```python
from build123d import *

# Parameters (mm, degrees)
F0_W     = 18
F0_H     = 18
F1_DEPTH = 2
F3_D     = 2.54
F5_D     = 2.54


with BuildPart() as f1:
    # F0 (on Top) → F1 (new body)
    with BuildSketch(Plane.XY):
        Rectangle(F0_W, F0_H)
    extrude(amount=F1_DEPTH)

    # F3 (through all)
    with Locations(Plane.XY.offset(2)):
        with Locations((6.7902, 6.7902)):
            Hole(F3_D / 2)

    # F5 (through all)
    with Locations(Plane(origin=(0, 0, 0), x_dir=(1, 0, 0), z_dir=(0, 0, -1))):
        with Locations((-6.7902, -6.7902)):
            Hole(F5_D / 2)


solid = f1.part
```
Model file for the job. Use its own axes, mm. Coordinates: 2 decimals unless noted, no trailing zeros. Loops run counter-clockwise (first coordinate to the right, second up) from the corner with the lowest first, then second, coordinate; pieces in that order, holes last. Notation, with made-up numbers: M -33,58 L -26,58 A35 ccw -26,90 Z; hole C -40,68 d9. An arc over 180 degrees is marked long. Use CSV: the item, a comma, the result in double quotes. Start each with the question number.
1. Band-saw the part on B-B, the plane z = 1.65. List the corners of the cut face in (x, y), then the cut area to 3 significant figures.
2. Flat gauge pin, fed straight in: pin 1 (2 mm diameter, centred on x = 6.79, y = 6.79, fed in from -Z). Where does the tip first touch, or does it go through?
3. Band-saw the part on A-A, the plane y = 7.75. List the corners of the cut face in (x, z).
4. Probe probe 1 along Y at (x, z) = (-6.75, 1.3); probe 2 along Y at (x, z) = (7.25, 1.45); probe 3 along X at (y, z) = (6.5, 0.7). List the from-to ranges inside material, lowest first. Write a range as [from, to].
5. Two-plate mould, pull along X, no slides. Class faces 1 (the cylindrical face through (-7.376, 7.917, 1.014)), 2 (the cylindrical face through (6.107, 7.861, 0.986)), 3 (the flat face through (0, 0, 2)), 4 (the flat face through (-9, 0, 1)): pulls with the +X half, pulls with the -X half, needs draft (parallel to the pull), parting line crosses it, or undercut.
Entries:
1,outline,"M -9,-9 L 9,-9 L 9,9 L -9,9 Z; hole C -6.79,6.79 d2.54; hole C 6.79,6.79 d2.54"
1,area,"314 mm2"
2,pin 1,"passes through"
3,outline,"M -9,0 L -7.62,0 L -7.62,2 L -9,2 Z; M -5.96,0 L 5.96,0 L 5.96,2 L -5.96,2 Z; M 7.62,0 L 9,0 L 9,2 L 7.62,2 Z"
4,probe 1,"y = [-9, 5.52], [8.06, 9]"
4,probe 2,"y = [-9, 5.61], [7.97, 9]"
4,probe 3,"x = [-9, -8.03], [-5.55, 5.55], [8.03, 9]"
5,face 1,"undercut"
5,face 2,"undercut"
5,face 3,"needs draft"
5,face 4,"pulls with the -X half"
